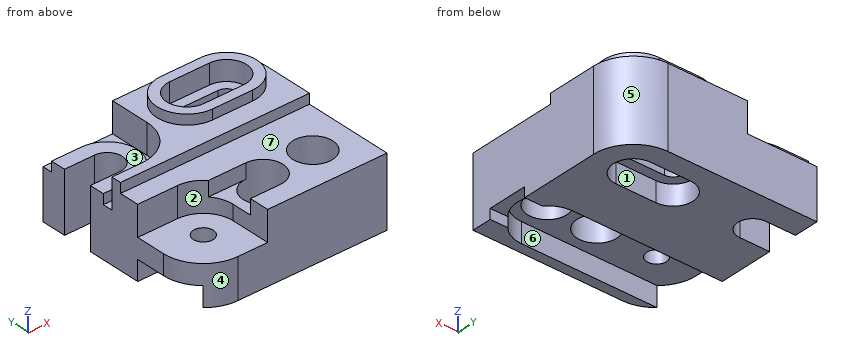
```python
from build123d import *

# Parameters (mm, degrees)
SKETCH1_W           = 190
SKETCH1_H           = 180
BOSS_EXTRUDE1_DEPTH = 70
CUT_EXTRUDE1_DEPTH  = 70
CUT_EXTRUDE2_DEPTH  = 20
CUT_EXTRUDE4_DEPTH  = 116
CUT_EXTRUDE5_DEPTH  = 116
SKETCH6_W           = 20
SKETCH6_H           = 90
CUT_EXTRUDE6_DEPTH  = 242
BOSS_EXTRUDE2_DEPTH = 10
CUT_EXTRUDE12_DEPTH = 20
BOSS_EXTRUDE4_DEPTH = 10
BOSS_EXTRUDE5_DEPTH = 30
CUT_EXTRUDE13_DEPTH = 10
SKETCH15_W          = 190
SKETCH15_H          = 10
BOSS_EXTRUDE6_DEPTH = 30
CUT_EXTRUDE14_DEPTH = 30
BOSS_EXTRUDE7_DEPTH = 30
BOSS_EXTRUDE8_DEPTH = 10
CUT_EXTRUDE15_DEPTH = 20
CUT_EXTRUDE16_DEPTH = 62
CUT_EXTRUDE17_DEPTH = 30
CUT_EXTRUDE18_DEPTH = 15
SKETCH25_R          = 20
CUT_EXTRUDE19_DEPTH = 50
SKETCH26_R          = 10
CUT_EXTRUDE20_DEPTH = 20
CUT_EXTRUDE21_DEPTH = 20
SKETCH28_W          = 10
SKETCH28_H          = 40
CUT_EXTRUDE22_DEPTH = 59


with BuildPart() as part:
    # Sketch1 → Boss-Extrude1 (new body)
    with BuildSketch(Plane.XY):
        with Locations((95, 90)):
            Rectangle(SKETCH1_W, SKETCH1_H)
    extrude(amount=BOSS_EXTRUDE1_DEPTH)

    # Sketch2 → Cut-Extrude1 (cut)
    with BuildSketch(Plane(origin=(0, 0, 0), x_dir=(-1, 0, 0), z_dir=(0, 0, -1))):
        with BuildLine():
            Line((-150, 150), (-110, 150))
            ThreePointArc((-110, 150), (-100, 140), (-110, 130))
            Line((-110, 130), (-150, 130))
            ThreePointArc((-150, 130), (-160, 140), (-150, 150))
        make_face()
    extrude(amount=-CUT_EXTRUDE1_DEPTH, mode=Mode.SUBTRACT)

    # Sketch3 → Cut-Extrude2 (cut)
    with BuildSketch(Plane(origin=(0, 0, 0), x_dir=(-1, 0, 0), z_dir=(0, 0, -1))):
        with BuildLine():
            Line((-110, 120), (-150, 120))
            ThreePointArc((-150, 120), (-170, 140), (-150, 160))
            Line((-150, 160), (-110, 160))
            ThreePointArc((-110, 160), (-90, 140), (-110, 120))
        make_face()
    extrude(amount=-CUT_EXTRUDE2_DEPTH, mode=Mode.SUBTRACT)

    # Sketch4 → Cut-Extrude4 (cut)
    with BuildSketch(Plane.XY.offset(70)):
        with BuildLine():
            Line((150, 180), (190, 180))
            Line((190, 180), (190, 140))
            ThreePointArc((190, 140), (178.284271247, 168.284271247), (150, 180))
        make_face()
        with BuildLine():
            Line((0, 40), (0, 0))
            Line((0, 0), (40, 0))
            ThreePointArc((40, 0), (11.715728753, 11.715728753), (0, 40))
        make_face()
    extrude(amount=-CUT_EXTRUDE4_DEPTH, mode=Mode.SUBTRACT)

    # Sketch5 → Cut-Extrude5 (cut)
    with BuildSketch(Plane.XY.offset(70)):
        with BuildLine():
            Line((30, 155), (0, 155))
            Line((0, 155), (0, 125))
            Line((0, 125), (30, 125))
            ThreePointArc((30, 125), (45, 140), (30, 155))
        make_face()
    extrude(amount=-CUT_EXTRUDE5_DEPTH, mode=Mode.SUBTRACT)

    # Sketch6 → Cut-Extrude6 (cut)
    with BuildSketch(Plane.ZY):
        with Locations((60, 135)):
            Rectangle(SKETCH6_W, SKETCH6_H)
    extrude(amount=-CUT_EXTRUDE6_DEPTH, mode=Mode.SUBTRACT)

    # Sketch7 → Boss-Extrude2 (add)
    with BuildSketch(Plane.XY.offset(50)):
        with BuildLine():
            Line((150, 110), (110, 110))
            ThreePointArc((110, 110), (80, 140), (110, 170))
            Line((110, 170), (150, 170))
            ThreePointArc((150, 170), (180, 140), (150, 110))
        make_face()
    extrude(amount=BOSS_EXTRUDE2_DEPTH)

    # Sketch11 → Cut-Extrude12 (cut)
    with BuildSketch(Plane(origin=(0, 0, 50), x_dir=(-1, 0, 0), z_dir=(0, 0, -1))):
        with BuildLine():
            Line((-150, 150), (-110, 150))
            ThreePointArc((-110, 150), (-100, 140), (-110, 130))
            Line((-110, 130), (-150, 130))
            ThreePointArc((-150, 130), (-160, 140), (-150, 150))
        make_face()
    extrude(amount=-CUT_EXTRUDE12_DEPTH, mode=Mode.SUBTRACT)

    # Sketch12 → Boss-Extrude4 (add)
    with BuildSketch(Plane.XY.offset(50)):
        with BuildLine():
            Line((30, 155), (0, 155))
            Line((0, 155), (0, 170))
            Line((0, 170), (30, 170))
            ThreePointArc((30, 170), (60, 140), (30, 110))
            Line((30, 110), (0, 110))
            Line((0, 110), (0, 125))
            Line((0, 125), (30, 125))
            ThreePointArc((30, 125), (45, 140), (30, 155))
        make_face()
    extrude(amount=BOSS_EXTRUDE4_DEPTH)

    # Sketch13 → Boss-Extrude5 (add)
    with BuildSketch(Plane.XY.offset(50)):
        with BuildLine():
            Line((150, 180), (0, 180))
            Line((0, 180), (0, 170))
            Line((0, 170), (30, 170))
            ThreePointArc((30, 170), (60, 140), (30, 110))
            Line((30, 110), (0, 110))
            Line((0, 110), (0, 100))
            Line((0, 100), (190, 100))
            Line((190, 100), (190, 140))
            ThreePointArc((190, 140), (178.284271247, 168.284271247), (150, 180))
        make_face()
        with BuildLine():
            ThreePointArc((110, 110), (80, 140), (110, 170))
            Line((110, 170), (150, 170))
            ThreePointArc((150, 170), (180, 140), (150, 110))
            Line((150, 110), (110, 110))
        make_face(mode=Mode.SUBTRACT)
    extrude(amount=BOSS_EXTRUDE5_DEPTH)

    # Sketch14 → Cut-Extrude13 (cut)
    with BuildSketch(Plane.XY.offset(60)):
        with BuildLine():
            Line((110, 170), (150, 170))
            ThreePointArc((150, 170), (180, 140), (150, 110))
            Line((150, 110), (110, 110))
            ThreePointArc((110, 110), (80, 140), (110, 170))
        make_face()
    extrude(amount=-CUT_EXTRUDE13_DEPTH, mode=Mode.SUBTRACT)

    # Sketch15 → Boss-Extrude6 (add)
    with BuildSketch(Plane.XY.offset(50)):
        with Locations((95, 95)):
            Rectangle(SKETCH15_W, SKETCH15_H)
    extrude(amount=BOSS_EXTRUDE6_DEPTH)

    # Sketch16 → Cut-Extrude14 (cut)
    with BuildSketch(Plane.XY.offset(80)):
        with BuildLine():
            Line((0, 180), (0, 170))
            Line((0, 170), (30, 170))
            ThreePointArc((30, 170), (60, 140), (30, 110))
            Line((30, 110), (0, 110))
            Line((0, 110), (0, 100))
            Line((0, 100), (30, 100))
            ThreePointArc((30, 100), (58.284271247, 111.715728753), (70, 140))
            Line((70, 140), (70, 180))
            Line((70, 180), (0, 180))
        make_face()
    extrude(amount=-CUT_EXTRUDE14_DEPTH, mode=Mode.SUBTRACT)

    # Sketch18 → Boss-Extrude7 (add)
    with BuildSketch(Plane.XY.offset(50)):
        with BuildLine():
            Line((150, 110), (110, 110))
            ThreePointArc((110, 110), (80, 140), (110, 170))
            Line((110, 170), (150, 170))
            ThreePointArc((150, 170), (180, 140), (150, 110))
        make_face()
    extrude(amount=BOSS_EXTRUDE7_DEPTH)

    # Sketch20 → Boss-Extrude8 (add)
    with BuildSketch(Plane.XY.offset(80)):
        with BuildLine():
            Line((110, 170), (150, 170))
            ThreePointArc((150, 170), (180, 140), (150, 110))
            Line((150, 110), (110, 110))
            ThreePointArc((110, 110), (80, 140), (110, 170))
        make_face()
    extrude(amount=BOSS_EXTRUDE8_DEPTH)

    # Sketch21 → Cut-Extrude15 (cut)
    with BuildSketch(Plane.XY.offset(90)):
        with BuildLine():
            Line((110, 160), (150, 160))
            ThreePointArc((150, 160), (170, 140), (150, 120))
            Line((150, 120), (110, 120))
            ThreePointArc((110, 120), (90, 140), (110, 160))
        make_face()
    extrude(amount=-CUT_EXTRUDE15_DEPTH, mode=Mode.SUBTRACT)

    # Sketch22 → Cut-Extrude16 (cut)
    with BuildSketch(Plane(origin=(0, 0, 50), x_dir=(-1, 0, 0), z_dir=(0, 0, -1))):
        with BuildLine():
            Line((-150, 150), (-110, 150))
            ThreePointArc((-110, 150), (-100, 140), (-110, 130))
            Line((-110, 130), (-150, 130))
            ThreePointArc((-150, 130), (-160, 140), (-150, 150))
        make_face()
    extrude(amount=-CUT_EXTRUDE16_DEPTH, mode=Mode.SUBTRACT)

    # Sketch23 → Cut-Extrude17 (cut)
    with BuildSketch(Plane.XY.offset(70)):
        with BuildLine():
            Line((0, 40), (0, 70))
            Line((0, 70), (40, 70))
            ThreePointArc((40, 70), (61.213203436, 61.213203436), (70, 40))
            Line((70, 40), (70, 0))
            Line((70, 0), (40, 0))
            ThreePointArc((40, 0), (11.715728753, 11.715728753), (0, 40))
        make_face()
    extrude(amount=-CUT_EXTRUDE17_DEPTH, mode=Mode.SUBTRACT)

    # Sketch24 → Cut-Extrude18 (cut)
    with BuildSketch(Plane.XY.offset(70)):
        with BuildLine():
            ThreePointArc((100, 20), (80, 40), (100, 60))
            Line((100, 60), (62.360679775, 60))
            ThreePointArc((62.360679775, 60), (68.025170769, 50.704662693), (70, 40))
            Line((70, 40), (70, 20))
            Line((70, 20), (100, 20))
        make_face()
    extrude(amount=-CUT_EXTRUDE18_DEPTH, mode=Mode.SUBTRACT)

    # Sketch25 → Cut-Extrude19 (cut)
    with BuildSketch(Plane.XY.offset(70)):
        with Locations((100, 40)):
            Circle(SKETCH25_R)
        with Locations((150, 40)):
            Circle(SKETCH25_R)
    extrude(amount=-CUT_EXTRUDE19_DEPTH, mode=Mode.SUBTRACT)

    # Sketch26 → Cut-Extrude20 (cut)
    with BuildSketch(Plane.XY.offset(40)):
        with Locations((40, 40)):
            Circle(SKETCH26_R)
    extrude(amount=-CUT_EXTRUDE20_DEPTH, mode=Mode.SUBTRACT)

    # Sketch27 → Cut-Extrude21 (cut)
    with BuildSketch(Plane(origin=(0, 0, 0), x_dir=(-1, 0, 0), z_dir=(0, 0, -1))):
        with BuildLine():
            Line((0, 40), (0, 70))
            Line((0, 70), (-150, 70))
            ThreePointArc((-150, 70), (-180, 40), (-150, 10))
            Line((-150, 10), (-13.542486889, 10))
            ThreePointArc((-13.542486889, 10), (-3.542486889, 23.542486889), (0, 40))
        make_face()
    extrude(amount=-CUT_EXTRUDE21_DEPTH, mode=Mode.SUBTRACT)

    # Sketch28 → Cut-Extrude22 (cut)
    with BuildSketch(Plane(origin=(190, 0, 0), x_dir=(0, 0, -1), z_dir=(1, 0, 0))):
        with Locations((-5, 40)):
            Rectangle(SKETCH28_W, SKETCH28_H)
    extrude(amount=-CUT_EXTRUDE22_DEPTH, mode=Mode.SUBTRACT)


solid = part.part
```
Design review of the part built by this model. Coordinates are the model's own, in mm. Face numbers are marked on the shaded views. A direction names the side the tool comes from. Coordinates: 2 decimals unless noted, no trailing zeros. Write each loop counter-clockwise with the first axis right and the second up, starting at its lowest first coordinate (ties: lowest second). Pieces come first, ordered by that corner, then holes. Notation, with made-up numbers: M 80,83 L 136,83 A17 cw 136,101 Z; hole C 10.25,-7 d11. An arc over 180 degrees is marked long. Answer as a JSON object with one key per item and string values.
Item 1: Add section B-B, the plane y = 16. Give the boundary of the cut face in (x, z).
Outcome:
{"outline": "M 8,20 L 168,20 L 168,0 L 190,0 L 190,70 L 70,70 L 70,40 L 8,40 Z"}
Item 2: Add section C-C, the plane x = 133. State how many separate pieces and enclosed holes the cut face has, and give its area (3 significant figures).
Outcome:
{"separate pieces": "3", "enclosed holes": "0", "area": "9,250 mm²"}
Item 3: Draft analysis for pull direction Y (two halves, no side actions). For the marked faces 4, 5, 6 and 7, state which applies: pulls with the +Y half, pulls with the -Y half, needs draft (parallel to the pull), parting line crosses it, or undercut.
Outcome:
{"face 4": "pulls with the -Y half", "face 5": "pulls with the +Y half", "face 6": "undercut", "face 7": "needs draft"}
Item 4: Insertion check: pin 1 Ø3 at (x, z) = (27, 28) entering from -Y; pin 2 Ø9 at (x, z) = (25, 54.5) entering from -Y; pin 3 Ø3 at (x, z) = (12, 56) entering from +Y. Each pin has a flat end and moves straight along its axis. Give the tip position at first contact, or say it passes through.
Outcome:
{"pin 1": "y = 1.69", "pin 2": "y = 70", "pin 3": "y = 170"}
Item 5: Add section A-A, the plane z = 66.5. Give the boundary of the cut face in (x, y).
Outcome:
{"outline": "M 0,70 L 40,70 A30 cw 62.36,60 L 100,60 A20 cw 100,20 L 70,20 L 70,0 L 190,0 L 190,140 A40 ccw 150,180 L 70,180 L 70,140 A40 cw 30,100 L 0,100 Z; hole M 110,130 L 150,130 A10 ccw 150,150 L 110,150 A10 ccw Z; hole C 150,40 d40"}
Item 6: Wall thickness on probe 1 along Y at (x, z) = (148, 84); probe 2 along Y at (x, z) = (150, 31); probe 3 along X at (y, z) = (33, 21.5) (3 decimals): over which ranges is each line inside the solid? List them lowest first.
Outcome:
{"probe 1": "110 to 120, 160 to 170", "probe 2": "0 to 20, 60 to 130, 150 to 180", "probe 3": "0.617 to 32.859, 47.141 to 81.265, 118.735 to 131.265, 168.735 to 190"}
Item 7: Machinability: for the marked faces 1, 2 and 3, which of the approach directions +Z, -Z, +X, -X, +Y, -Y give a long, thin tool a straight path to every point of the face, cutting with its end or side? Answer none if there is none.
Outcome:
{"face 1": "-Z", "face 2": "+Z, -X, -Y", "face 3": "+Z, -X, +Y"}
